Work out the finished part from the listing and answer in its coordinate system (mm). A direction names the side the tool comes from. Round coordinates to 2 decimals unless told otherwise and drop trailing zeros. Order: outer loops, then holes, each group sorted by start corner. A loop starts at its lowest first (then second) coordinate and runs counter-clockwise, first axis right, second up. Notation, with made-up numbers: (52, 76.25) - (72, 76.25) arc R27 cw to (72, 99.25) - close; hole circle Ø11 at (0, 18.5). An arc over 180 degrees is marked (long way). Use one line per item in the form item = value. Start each with the question number.
Q1. The part is cut by section B-B on y = 4. Determine the outline of the cut face in (x, z).
Q2. Find the intervals of material crossed by line 1 (Z direction, x = 17.5, y = 3.5); line 2 (X direction, y = 34, z = 16.5); line 3 (Y direction, x = 20, z = 3), in increasing order. Write a range as [from, to].
Q3. The part is cut by section D-D on z = -11. Determine the outline of the cut face in (x, y).
Q4. Given P1, Ø4, axis at y = -36, z = 6.5, coming from the +X side; P2, Ø4, axis at x = 33, z = 7.5, coming from the +Y side; P3, Ø7, axis at x = -77, y = -36, coming from the -Z side; P4, Ø20, axis at x = 30.11, y = 6.76, coming from the +Z side, each flat-ended and moving along its own axis, determine where each tip first touches the part or whether it passes through.
Q5. Which of the six approach directions +Z, -Z, +X, -X, +Y, -Y give full straight-line access (tool end or side, diameter ignored) to faces 1 (the flat face through (-85.728, -38, 8)), 2 (the flat face through (-61.953, -32, -8)), 3 (the flat face through (-22.13, -56.56, 1.48)), 4 (the cylindrical face through (80.268, 17.017, 13.414)), 5 (the flat face through (-34, -57, 0))?
Q6. For a pull along Y with two mould halves and no side action, classify faces 6 (the flat face through (-74, -33, 1.5)), 7 (the flat face through (-20.7, -59.2, 1.5)), 8 (the cylindrical face through (88.5, 15.08, 0.35)), 9 (the flat face through (95, 48, 1.5)) as +Y half, -Y half, draft (parallel to the pull), parting line (faces both ways), or undercut.
Q7. The part is cut by section C-C on x = 31.5. Determine the outline of the cut face in (y, z).
from build123d import *

# Parameters (mm, degrees)
ESTRUSIONE_ESTRUSIONE1_DEPTH = 15
TAGLIO_ESTRUSIONE1_DEPTH     = 13.5
SCHIZZO3_R                   = 15
SCHIZZO3_R_2                 = 13
SCHIZZO3_R_3                 = 11
SCHIZZO3_R_4                 = 9
TAGLIO_ESTRUSIONE2_DEPTH     = 17.5
ESTRUSIONE_ESTRUSIONE3_DEPTH = 25
TAGLIO_ESTRUSIONE4_DEPTH     = 23.5
TAGLIO_ESTRUSIONE5_DEPTH     = 23.5
TAGLIO_ESTRUSIONE6_DEPTH     = 27.5
ESTRUSIONE_SOTTILE2_START    = -15
ESTRUSIONE_SOTTILE2_DEPTH    = 30
ESTRUSIONE_ESTRUSIONE4_DEPTH = 1.5
ESTRUSIONE_SOTTILE3_DEPTH    = 3


with BuildPart() as part:
    # Schizzo1 → Estrusione-Estrusione1 (new body, symmetric)
    with BuildSketch(Plane.XY):
        Polygon((-61.953104657, -55.142919533), (-61.953104657, -5.142919533), (88.046895343, 44.857080467), (88.046895343, 14.857080467), align=None)
    extrude(amount=ESTRUSIONE_ESTRUSIONE1_DEPTH, both=True)

    # Schizzo2 → Taglio-Estrusione1 (cut)
    with BuildSketch(Plane.XY.offset(15)):
        Polygon((85.046895343, 16.767669539), (85.046895343, 40.694802807), (-58.953104657, -7.305197193), (-58.953104657, -50.432330461), align=None)
    taglio_estrusione1 = extrude(amount=-TAGLIO_ESTRUSIONE1_DEPTH, mode=Mode.SUBTRACT)

    # Specchia1: Taglio-Estrusione1 across plane
    add(taglio_estrusione1.mirror(Plane.XY), mode=Mode.SUBTRACT)

    # Schizzo3 → Taglio-Estrusione2 (cut, through all)
    with BuildSketch(Plane.XY.offset(1.5)):
        with Locations((-33.953104657, -18.868763827)):
            Circle(SCHIZZO3_R)
        with Locations((-1.456420476, -5.870090155)):
            Circle(SCHIZZO3_R_2)
        with Locations((30.111787014, 6.757192842)):
            Circle(SCHIZZO3_R_3)
        with Locations((57.966087741, 17.898913132)):
            Circle(SCHIZZO3_R_4)
    extrude(amount=-TAGLIO_ESTRUSIONE2_DEPTH, mode=Mode.SUBTRACT)

    # Schizzo4 → Estrusione-Estrusione3 (add, symmetric)
    with BuildSketch(Plane.XY):
        with BuildLine():
            Line((70.629518485, 29.197898059), (81.478220515, 72.870608809))
            ThreePointArc((81.478220515, 72.870608809), (96.623057398, 81.988389009), (105.740837598, 66.843552126))
            Line((105.740837598, 66.843552126), (94.892135568, 23.170841376))
            ThreePointArc((94.892135568, 23.170841376), (79.747298685, 14.053061176), (70.629518485, 29.197898059))
        make_face()
    extrude(amount=ESTRUSIONE_ESTRUSIONE3_DEPTH, both=True)

    # Schizzo5 → Taglio-Estrusione4 (cut)
    with BuildSketch(Plane.XY.offset(25)):
        with BuildLine():
            Line((91.980621518, 23.894088178), (102.829323548, 67.566798928))
            ThreePointArc((102.829323548, 67.566798928), (95.899810596, 79.076874959), (84.389734565, 72.147362007))
            Line((84.389734565, 72.147362007), (73.541032535, 28.474651257))
            ThreePointArc((73.541032535, 28.474651257), (80.470545487, 16.964575226), (91.980621518, 23.894088178))
        make_face()
    extrude(amount=-TAGLIO_ESTRUSIONE4_DEPTH, mode=Mode.SUBTRACT)

    # Schizzo6 → Taglio-Estrusione5 (cut)
    with BuildSketch(Plane(origin=(0, 0, -25), x_dir=(-1, 0, 0), z_dir=(0, 0, -1))):
        with BuildLine():
            Line((-73.541032535, 28.474651257), (-84.389734565, 72.147362007))
            ThreePointArc((-84.389734565, 72.147362007), (-95.899810596, 79.076874959), (-102.829323548, 67.566798928))
            Line((-102.829323548, 67.566798928), (-91.980621518, 23.894088178))
            ThreePointArc((-91.980621518, 23.894088178), (-80.470545487, 16.964575226), (-73.541032535, 28.474651257))
        make_face()
    extrude(amount=-TAGLIO_ESTRUSIONE5_DEPTH, mode=Mode.SUBTRACT)

    # Schizzo7 → Taglio-Estrusione6 (cut, through all)
    with BuildSketch(Plane.XY.offset(1.5)):
        with BuildLine():
            Line((76.937798926, 27.630863321), (87.786500957, 71.303574071))
            ThreePointArc((87.786500957, 71.303574071), (95.056022661, 75.680108567), (99.432557157, 68.410586863))
            Line((99.432557157, 68.410586863), (88.583855126, 24.737876113))
            ThreePointArc((88.583855126, 24.737876113), (81.314333422, 20.361341617), (76.937798926, 27.630863321))
        make_face()
    extrude(amount=-TAGLIO_ESTRUSIONE6_DEPTH, mode=Mode.SUBTRACT)

    # Schizzo8 → Estrusione-Sottile2 (add)
    with BuildSketch(Plane.XY.offset(ESTRUSIONE_SOTTILE2_START)):
        Polygon((-61.953104657, -5.142919533), (-88.727527571, -14.067727171), (-88.727527571, -58.470604197), (-85.727527571, -58.470604197), (-85.727527571, -16.230004831), (-61.004421359, -7.988969427), align=None)
    extrude(amount=ESTRUSIONE_SOTTILE2_DEPTH)

    # Schizzo9 → Estrusione-Estrusione4 (add, symmetric)
    with BuildSketch(Plane.XY):
        Polygon((-85.727527571, -58.470604197), (-61.953104657, -55.142919533), (-61.953104657, -8.305197193), (-85.727527571, -16.230004831), align=None)
    extrude(amount=ESTRUSIONE_ESTRUSIONE4_DEPTH, both=True)

    # Schizzo11 → Estrusione-Sottile3 (add)
    with BuildSketch(Plane.XY):
        with BuildLine():
            Line((-33.953104657, -42.076252866), (-33.953104657, -55.795467437))
            ThreePointArc((-33.953104657, -55.795467437), (-32.101805724, -59.169350026), (-28.261562796, -59.420199997))
            Line((-28.261562796, -59.420199997), (-15.829441857, -53.618543559))
            Line((-15.829441857, -53.618543559), (-14.560785461, -56.337092979))
            Line((-14.560785461, -56.337092979), (-26.9929064, -62.138749417))
            ThreePointArc((-26.9929064, -62.138749417), (-33.713331525, -61.699761968), (-36.953104657, -55.795467437))
            Line((-36.953104657, -55.795467437), (-36.953104657, -42.076252866))
            Line((-36.953104657, -42.076252866), (-33.953104657, -42.076252866))
        make_face()
    extrude(amount=ESTRUSIONE_SOTTILE3_DEPTH)


solid = part.part
Found:
q1.outline = (-34.52, -15) - (-25.04, -15) - (-25.04, -1.5) - (-9.92, -1.5) - (-9.92, 1.5) - (-25.04, 1.5) - (-25.04, 15) - (-34.52, 15) - close; (7, -1.5) - (19.46, -1.5) - (19.46, 1.5) - (7, 1.5) - close; (40.76, -1.5) - (57.69, -1.5) - (57.69, -15) - (64.78, -15) - (64.78, 15) - (57.69, 15) - (57.69, 1.5) - (40.76, 1.5) - close
q2.line_1 = [-1.5, 1.5]
q2.line_2 = [71.82, 74.91], [94.49, 97.58]
q2.line_3 = [-16.9, -13.59], [19.01, 22.17]
q3.outline = (-88.73, -58.47) - (-85.73, -58.47) - (-85.73, -16.23) - (-61.95, -8.31) - (-61.95, -55.14) - (88.05, 14.86) arc R12.5 ccw to (94.89, 23.17) - (105.74, 66.84) arc R12.5 ccw to (81.48, 72.87) - (73.3, 39.94) - (-88.73, -14.07) - close; hole (-58.95, -50.43) - (79.42, 14.14) arc R12.5 cw to (70.63, 29.2) - (72.44, 36.49) - (-58.95, -7.31) - close; hole (73.54, 28.47) arc R9.5 ccw to (91.98, 23.89) - (102.83, 67.57) arc R9.5 ccw to (84.39, 72.15) - close
q4.P1 = -16.65
q4.P2 = 27.17
q4.P3 = -1.5
q4.P4 = through
q5.face_1 = +Z, -Y
q5.face_2 = -Z, -Y
q5.face_3 = +Z, -Z
q5.face_4 = +Z
q5.face_5 = -Z, +X, -Y
q6.face_6 = draft
q6.face_7 = -Y half
q6.face_8 = undercut
q6.face_9 = undercut
q7.outline = (-11.53, -15) - (-8.22, -15) - (-8.22, -1.5) - (-4.15, -1.5) - (-4.15, 1.5) - (-8.22, 1.5) - (-8.22, 15) - (-11.53, 15) - close; (17.67, -1.5) - (22.85, -1.5) - (22.85, -15) - (26.01, -15) - (26.01, 15) - (22.85, 15) - (22.85, 1.5) - (17.67, 1.5) - close
